```python
from build123d import *

# Parameters (mm, degrees)
BOSS_EXTRUDE1_DEPTH = 19.05
SKETCH2_R           = 1.5875
SKETCH2_R_2         = 1.5874999999999988
CUT_EXTRUDE1_DEPTH  = 19.05
CUT_EXTRUDE2_DEPTH  = 6.35
FILLET1_R           = 1.27
SKETCH3_R           = 1.3523393116529026
BOSS_EXTRUDE2_DEPTH = 2.54
FILLET2_R           = 0.762
SKETCH4_R           = 0.6365323226185287
CUT_EXTRUDE3_DEPTH  = 50.150613196033525


with BuildPart() as part:
    # Sketch1 → Boss-Extrude1 (new body)
    with BuildSketch(Plane(origin=(0, 0, 0), x_dir=(0, 0, -1), z_dir=(1, 0, 0))):
        with BuildLine():
            Line((-4.7625, 0), (-4.7625, 44.8056))
            ThreePointArc((-4.7625, 44.8056), (2.9e-16, 49.5681), (4.7625, 44.8056))
            Line((4.7625, 44.8056), (4.762500000000005, 5.8e-16))
            ThreePointArc((4.762500000000005, 5.8e-16), (1.35e-15, -4.762500000000005), (-4.7625, 0))
        make_face()
    extrude(amount=BOSS_EXTRUDE1_DEPTH)

    # Sketch2 → Cut-Extrude1 (cut)
    with BuildSketch(Plane(origin=(19.05, 0, 0), x_dir=(0, 0, -1), z_dir=(1, 0, 0))):
        Circle(SKETCH2_R)
        with Locations((0, 44.8056)):
            Circle(SKETCH2_R_2)
    extrude(amount=-CUT_EXTRUDE1_DEPTH, mode=Mode.SUBTRACT)

    # 3DSketch1 → Cut-Extrude2 (cut, symmetric)
    with BuildSketch(Plane(origin=(9.524999999999954, 44.80559999999997, -4.762500000000004), x_dir=(0, -0.9781419365644765, 0.20793833685469326), z_dir=(-1, -9.3e-16, 3.6e-16))):
        with BuildLine():
            Line((0, 0), (9.316801945776646, -1.9806126585409503))
            ThreePointArc((9.316801945776646, -1.9806126585409503), (5.6487073021588, 3.668094643617845), (11.2974146043176, 7.336189287235693))
            Line((11.2974146043176, 7.336189287235693), (1.9806126585409412, 9.316801945776648))
            ThreePointArc((1.9806126585409412, 9.316801945776648), (-3.6680946436178474, 5.648707302158794), (0, 0))
        make_face()
        with BuildLine():
            Line((45.806849011474235, 0), (36.49004706569759, 1.980612658540955))
            ThreePointArc((36.49004706569759, 1.980612658540955), (40.15814170931544, -3.668094643617836), (34.50943440715664, -7.336189287235687))
            Line((34.50943440715664, -7.336189287235687), (43.82623635293327, -9.316801945776637))
            ThreePointArc((43.82623635293327, -9.316801945776637), (49.47494365509206, -5.648707302158793), (45.806849011474235, 0))
        make_face()
    extrude(amount=CUT_EXTRUDE2_DEPTH, both=True, mode=Mode.SUBTRACT)

    # Fillet1
    fillet1_edges = [part.edges().sort_by_distance(p)[0] for p in [
        (19.05, 49.5681, 7e-17),
        (19.05, 22.4028, 4.7625),
        (15.874999999999961, 40.04309999999998, 4.762500000000003),
        (15.874999999999957, 40.043099999999974, -4.762500000000005),
        (3.174999999999959, 40.04309999999996, -4.762499999999999),
        (3.1749999999999625, 40.04309999999997, 4.762500000000008),
        (19.05, -4.762500000000005, -2.98e-15),
        (0, 22.4028, 4.7625),
        (0, 49.5681, 7e-17),
        (15.874999999999995, 4.762500000000003, 4.762499999999996),
        (15.874999999999991, 4.762500000000003, -4.762500000000006),
        (3.1749999999999954, 4.762499999999989, 4.762500000000001),
        (3.174999999999992, 4.762499999999989, -4.762500000000001),
        (0, 22.4028, -4.762500000000003),
        (0, -4.762500000000005, -2.98e-15),
        (19.05, 22.4028, -4.762500000000003),
    ]]
    fillet(fillet1_edges, radius=FILLET1_R)

    # Sketch3 → Boss-Extrude2 (add)
    with BuildSketch(Plane.ZY):
        with Locations((-2.068463746823568, 42.49092897757123)):
            Circle(SKETCH3_R)
    extrude(amount=BOSS_EXTRUDE2_DEPTH)

    # Fillet2
    fillet2_edges = [part.edges().sort_by_distance(p)[0] for p in [
        (-2.54, 42.49092897757123, -3.42080305847647),
    ]]
    fillet(fillet2_edges, radius=FILLET2_R)

    # Sketch4 → Cut-Extrude3 (cut, through all)
    with BuildSketch(Plane(origin=(0, 10.403230824440865, 18.01892435079848), x_dir=(-1, 0, 0), z_dir=(0, 0.49999999999999484, 0.8660254037844416))):
        with Locations(Location((0.8782218587697344, -37.93359892462922, 0), (0, 0, 90))):
            Circle(SKETCH4_R)
    extrude(amount=-CUT_EXTRUDE3_DEPTH, mode=Mode.SUBTRACT)


solid = part.part
```
Part model, mm, in its own coordinate system. A direction names the side the tool comes from. Round coordinates to 2 decimals unless told otherwise and drop trailing zeros. Write each loop counter-clockwise with the first axis right and the second up, starting at its lowest first coordinate (ties: lowest second). Pieces come first, ordered by that corner, then holes.
Item 1: Cut at A-A, the plane y = 20.5. Give the cut face in (x, z), plus the area to 3 significant figures.
Results:
outline: (0, -3.49) arc R1.27 ccw to (1.27, -4.76) - (17.78, -4.76) arc R1.27 ccw to (19.05, -3.49) - (19.05, 3.49) arc R1.27 ccw to (17.78, 4.76) - (1.27, 4.76) arc R1.27 ccw to (0, 3.49) - close
area: 180 mm2
Item 2: Cut at B-B, the plane z = 0. Count the separate pieces of the cut face and the enclosed holes in it, plus the area to 3 significant figures.
Results:
separate pieces: 5
enclosed holes: 0
area: 750 mm2
Item 3: Probe L1, parallel to Y at x = 17.6, z = 0; L2, parallel to X at y = 46.5, z = -0.25 (3 decimals); L3, parallel to Y at x = 0.7, z = 0. List the from-to ranges inside material, lowest first.
Results:
L1: y = -4.76 to -1.59, 1.59 to 43.22, 46.39 to 49.57
L2: x = 0 to 3.175, 15.875 to 19.05
L3: y = -4.63 to -1.59, 1.59 to 43.22, 46.39 to 49.43
Item 4: Two-plate mould, pull along Z, no slides. Class faces 1 (the cylindrical face through (16.257, 3.771, 4.4)), 2 (the flat face through (3.175, 43, 0)), 3 (the cylindrical face through (-0.69, 42.06, -1.8)), 4 (the cylindrical face through (1.61, -1.55, 0.34)): +Z half, -Z half, draft (parallel to the pull), parting line (faces both ways), or undercut.
Results:
face 1: +Z half
face 2: draft
face 3: undercut
face 4: undercut
Item 5: Which spindle directions (+Z, -Z, +X, -X, +Y, -Y) get a long thin tool onto all of the face, cutting with end or side? Do faces 5 (the cylindrical face through (2.793, 3.771, 4.4)), 6 (the cylindrical face through (16.257, 41.035, -4.4)), 7 (the cylindrical face through (9.632, 40.042, -0.105)), 8 (the cylindrical face through (-0.88, 41.17, -2.36)). Say none if no direction does.
Results:
face 5: +Z, -Y
face 6: -Z, +Y
face 7: +Y
face 8: -X
Item 6: Cut at C-C, the plane x = 5.25. Give the cut face in (y, z) (1 decimal).
Results:
outline: (9.5, -4.8) - (35.3, -4.8) arc R4.8 ccw to (35.3, 4.8) - (9.5, 4.8) arc R4.8 ccw to start
Item 7: Drop flat-ended pins along their axis: pin 1 Ø3.5 at (y, z) = (0, 0) entering from +X; pin 2 Ø1.5 at (y, z) = (33, 3) entering from -X; pin 3 Ø1.5 at (x, z) = (9, 0) entering from -Y; pin 4 Ø1 at (x, z) = (8.5, 3) entering from +Y. Give the stop position or say it passes through.
Results:
pin 1: stops at x = 19.05
pin 2: stops at x = 0
pin 3: stops at y = 4.76
pin 4: stops at y = 39.33
